Geometry: final body of the model. Coordinates: model frame, mm. Face numbers are marked on the shaded views. A direction names the side the tool comes from. Give positions to 0.01 mm unless a question says otherwise; leave off trailing zeros. Order: outer loops, then holes, each group sorted by start corner. A loop starts at its lowest first (then second) coordinate and runs counter-clockwise, first axis right, second up. Notation, with made-up numbers: M 40.25,61.5 L 69.25,61.5 A14 ccw 69.25,88.5 Z; hole C 83,80.5 d11. An arc over 180 degrees is marked long. Write item = value, one per line. Start each with the question number.
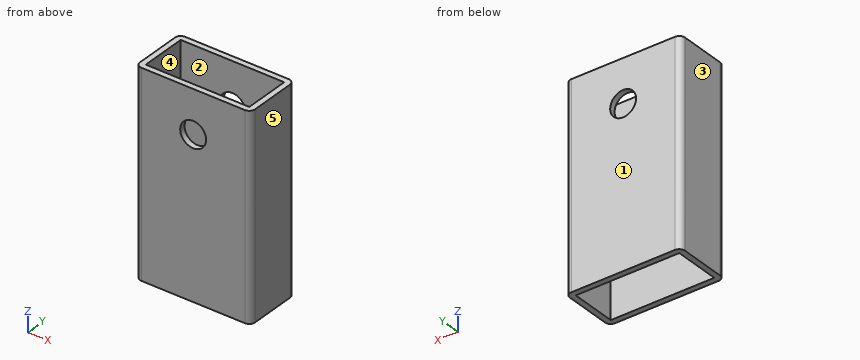
Autodesk Inventor part; units mm, degrees
ref_plane "YZ Plane" through (0, 0, 0) normal (1, 0, 0) x (0, 1, 0)
ref_plane "XZ Plane" through (0, 0, 0) normal (0, 1, 0) x (-1, 0, 0)
ref_plane "XY Plane" through (0, 0, 0) normal (0, 0, 1) x (1, 0, 0)
sketch "Sketch1" plane through (0, 0, 0) normal (0, 0, 1) x (1, 0, 0)
  line L0 (-20, 10) -> (20, 10)
  line L1 (20, 10) -> (20, -10)
  line L2 (20, -10) -> (-20, -10)
  line L3 (-20, -10) -> (-20, 10)
  line L4 (-20, 10) -> (20, -10) construction
  line L5 (20, 10) -> (-20, -10) construction
  line L6 (18, 8) -> (-18, 8)
  line L7 (-18, 8) -> (-18, -8)
  line L8 (-18, -8) -> (18, -8)
  line L9 (18, -8) -> (18, 8)
  point P0 (0, 0)
  dimension "d0" = 40
  dimension "d1" = 20
  dimension "d2" = 2
extrude "Extrusion1" add sketch "Sketch1" along normal mid plane 70
fillet "Fillet1" radius 2 4 edges at (-20, 10, 0) (-20, -10, 0) (20, -10, 0) (20, 10, 0)
sketch "Sketch4" plane through (0, 0, 0) normal (0, 1, 0) x (-1, 0, 0)
  line L0 (18, 35) -> (-18, 35)
  line L1 (-18, -35) -> (18, -35)
  circle A0 centre (0, 20) radius 4.5
  circle A1 centre (0, -20) radius 4.5
  line L2 (48.8004, 0) -> (-48.8004, 0) construction
  point P0 (0, 0)
  point P1 (0, 0)
  dimension "d20" = 9
  dimension "d21" = 15
extrude "Extrusion4" cut sketch "Sketch4" along normal through all both and the other way through all contours A0
properties part number "Leg tube 3"
1) Access query for the marked faces 1 and 2. Directions: +Z, -Z, +X, -X, +Y, -Y. A direction counts if a zero-diameter tool reaches every point of the face in a straight line with its end or side. Return the directions, or none.
2) Draft query along X for the marked faces 3, 4 and 5. Return one class per face: pulls with the +X half, pulls with the -X half, needs draft (parallel to the pull), parting line crosses it, or undercut.
3) Cut plane D-D (x = 0). Return loops of the section in (y, z), plus the area to 3 significant figures.
4) Cut plane A-A (y = 4.25). Return loops of the section in (x, z).
5) Cut plane C-C (x = 17). Return loops of the section in (y, z).
6) Cut plane B-B (z = 20). Return loops of the section in (x, y), plus the area to 3 significant figures.
7) Ray query, L1, parallel to Y at x = 15.5, z = -8; L2, parallel to X at y = 1.5, z = 14; L3, parallel to Z at x = 0, y = 8.7. Return the intervals inside material, ascending.
8) Pin query (flat end, axial travel): pin 1 Ø3 at (x, y) = (-6.5, -5) entering from -Z; pin 2 Ø10 at (x, y) = (14, 5.5) entering from +Z. Return the tip coordinate at first contact, or that it passes through.
Reply:
q1.face_1 = +Z, -Z, +X, -X, +Y
q1.face_2 = +Z, -Z
q2.face_3 = pulls with the -X half
q2.face_4 = undercut
q2.face_5 = pulls with the +X half
q3.outline = M -10,-35 L -8,-35 L -8,15.5 L -10,15.5 Z; M -10,24.5 L -8,24.5 L -8,35 L -10,35 Z; M 8,-35 L 10,-35 L 10,15.5 L 8,15.5 Z; M 8,24.5 L 10,24.5 L 10,35 L 8,35 Z
q3.area = 244 mm²
q4.outline = M -20,-35 L -18,-35 L -18,35 L -20,35 Z; M 18,-35 L 20,-35 L 20,35 L 18,35 Z
q5.outline = M -10,-35 L -8,-35 L -8,35 L -10,35 Z; M 8,-35 L 10,-35 L 10,35 L 8,35 Z
q6.outline = M -20,-8 A2 ccw -18,-10 L -4.5,-10 L -4.5,-8 L -18,-8 L -18,8 L -4.5,8 L -4.5,10 L -18,10 A2 ccw -20,8 Z; M 4.5,-10 L 18,-10 A2 ccw 20,-8 L 20,8 A2 ccw 18,10 L 4.5,10 L 4.5,8 L 18,8 L 18,-8 L 4.5,-8 Z
q6.area = 185 mm²
q7.L1 = -10 to -8, 8 to 10
q7.L2 = -20 to -18, 18 to 20
q7.L3 = -35 to 15.5, 24.5 to 35
q8.pin_1 = through
q8.pin_2 = 35
